from build123d import *

# Parameters (mm, degrees)
SKETCH_1_R        = 0.75
EXTRUDE_879_DEPTH = 0.8


with BuildPart() as part:
    # 草图1 → Extrude 879 (new body)
    with BuildSketch(Plane.XY):
        with BuildLine():
            Line((-1.385948162, -3.345974849), (-2.066490535, -4.988949476))
            ThreePointArc((-2.066490535, -4.988949476), (0, 5.4), (2.066490535, -4.988949476))
            Line((2.066490535, -4.988949476), (1.385948162, -3.345974849))
            ThreePointArc((1.385948162, -3.345974849), (1.591085636, -1.846752193), (2.997763625, -1.289072183))
            ThreePointArc((2.997763625, -1.289072183), (3.811994555, -1.04860419), (4.147928602, -0.268895796))
            ThreePointArc((4.147928602, -0.268895796), (0, 3.75), (-4.147928602, -0.268895796))
            ThreePointArc((-4.147928602, -0.268895796), (-3.811994555, -1.04860419), (-2.997763625, -1.289072183))
            ThreePointArc((-2.997763625, -1.289072183), (-1.591085636, -1.846752193), (-1.385948162, -3.345974849))
        make_face()
        with Locations((-2.84604621, -2.951274465)):
            Circle(SKETCH_1_R, mode=Mode.SUBTRACT)
        with Locations(Location((2.84604621, -2.951274465, 0), (0, 0, 180))):
            Circle(SKETCH_1_R, mode=Mode.SUBTRACT)
    extrude(amount=EXTRUDE_879_DEPTH)


solid = part.part
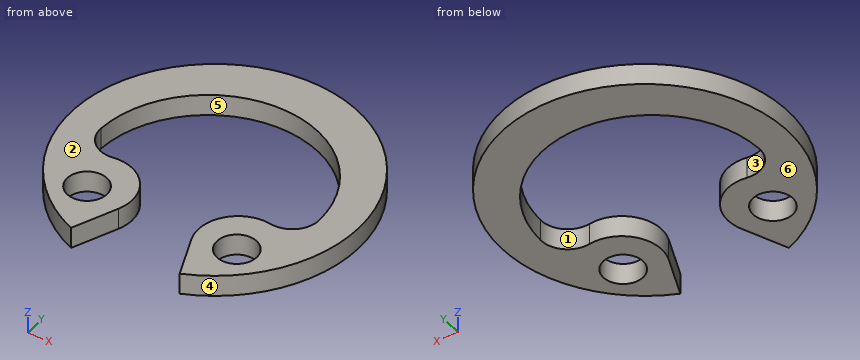
Check sheet for the modelled part. Datum: model origin and axes. Units: mm. Face numbers are marked on the shaded views. A direction names the side the tool comes from. Give positions to 0.01 mm unless a question says otherwise; leave off trailing zeros. Write each loop counter-clockwise with the first axis right and the second up, starting at its lowest first coordinate (ties: lowest second). Pieces come first, ordered by that corner, then holes. Notation, with made-up numbers: (57.5, -5.5) -> (105.5, -5.5) arc R21 cw to (105.5, 21.5) -> close; hole circle Ø6 at (24.5, 14). An arc over 180 degrees is marked (long way). One line per item, written item: value. Start each with the question number.
Item 1: Draft check along Y on the marked faces 1, 2, 3 and 4. Enter one of: +Y half, -Y half, draft (parallel to the pull), parting line (faces both ways), or undercut.
Item 2: Section check A-A on y = 2.5. Record the cut outline in (x, z), then the cut area to 3 significant figures.
Item 3: Material ranges on probe 1 along Y at (x, z) = (-3, 0.35); probe 2 along Y at (x, z) = (2.5, 0.75); probe 3 along X at (y, z) = (0.5, 0.65), recorded low to high. Write a range as from..to.
Item 4: Section check C-C on y = -0.5. Record the cut outline in (x, z).
Item 5: Section check D-D on x = 1. Record the cut outline in (y, z).
Item 6: Tool access check on the marked faces 5 and 6. Record the directions out of +Z, -Z, +X, -X, +Y, -Y that give a thin tool (end or side, any length) a straight path to the whole face; none if there is none.
Results list:
1. face 1: undercut
1. face 2: draft
1. face 3: undercut
1. face 4: parting line
2. outline: (-4.79, 0) -> (-2.97, 0) -> (-2.97, 0.8) -> (-4.79, 0.8) -> close; (2.97, 0) -> (4.79, 0) -> (4.79, 0.8) -> (2.97, 0.8) -> close
2. area: 2.91 mm²
3. probe 1: -4.49..-3.69, -2.22..-1.29, 2.47..4.49
3. probe 2: -4.79..-3.62, -2.29..-1.3, 2.91..4.79
3. probe 3: -5.38..-4.05, 4.05..5.38
4. outline: (-5.38, 0) -> (-4.13, 0) -> (-4.13, 0.8) -> (-5.38, 0.8) -> close; (4.13, 0) -> (5.38, 0) -> (5.38, 0.8) -> (4.13, 0.8) -> close
5. outline: (3.63, 0) -> (5.31, 0) -> (5.31, 0.8) -> (3.63, 0.8) -> close
6. face 5: +Z, -Z
6. face 6: -Z, +X, -X, +Y, -Y
